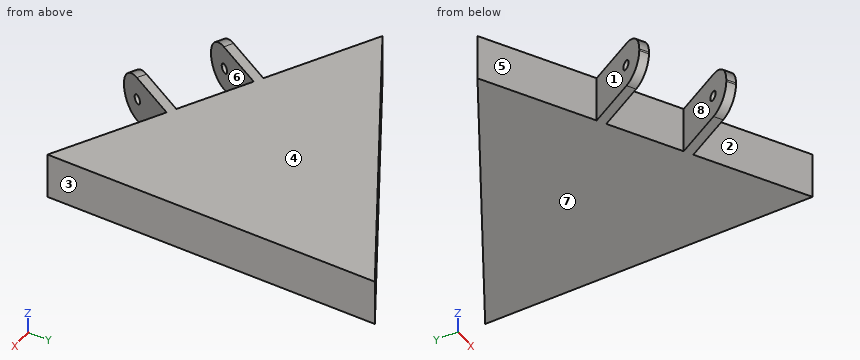
```python
from build123d import *

# Parameters (mm, degrees)
F1_DEPTH = 12.7
F2_W     = 2.54
F2_H     = 12.7
F3_DEPTH = 20.32
F4_R     = 1.27
F5_DEPTH = 39.1414
F6_R     = 6.096


with BuildPart() as f1:
    # F0 (on Top) → F1 (new body)
    with BuildSketch(Plane.XY):
        Polygon((25.4, -43.9940905122), (25.4, 43.9940905122), (-50.8, 0), align=None)
    extrude(amount=F1_DEPTH)

    # F2 (on face) → F3 (join)
    with BuildSketch(Plane(origin=(-12.7, -21.9970452561, 0), x_dir=(0.8660254038, -0.5, 0), z_dir=(-0.5, -0.8660254038, 0))):
        with Locations((11.43, 6.35)):
            Rectangle(F2_W, F2_H)
        with Locations((-11.43, 6.35)):
            Rectangle(F2_W, F2_H)
    extrude(amount=F3_DEPTH)

    # F4 (on face) → F5 (cut)
    with BuildSketch(Plane(origin=(10.9985226281, -6.35, 0), x_dir=(0.5, 0.8660254038, 0), z_dir=(0.8660254038, -0.5, 0))):
        with Locations((-39.37, 6.35)):
            Circle(F4_R)
    extrude(amount=-F5_DEPTH, mode=Mode.SUBTRACT)

    # F6
    f6_edges = [f1.edges().sort_by_distance(p)[0] for p in [
        (-32.75867, -33.879681, 0),
        (-32.75867, -33.879681, 12.7),
        (-12.96133, -45.309681, 12.7),
        (-12.96133, -45.309681, 0),
    ]]
    fillet(f6_edges, radius=F6_R)


solid = f1.part
```
The model under review builds one solid part; all positions refer to its coordinate system, in mm. Face numbers are marked on the shaded views. A direction names the side the tool comes from. Round coordinates to 2 decimals unless told otherwise and drop trailing zeros. Loops run counter-clockwise (first coordinate to the right, second up) from the corner with the lowest first, then second, coordinate; pieces in that order, holes last.
1) Clearance check with flat-ended pins moving along their axes: P1, Ø1.5, axis at y = -16.5, z = 4, coming from the -X side; P2, Ø5, axis at y = 25.5, z = 6.5, coming from the -X side; P3, Ø3, axis at x = -18, z = 5, coming from the +Y side. State where each tip first meets the part, or that it passes through.
Values follow:
P1: stops at x = -24.62
P2: stops at x = -10.96
P3: stops at y = 19.8
2) The part is to be moulded in two halves that separate along X. For the marked faces 1, 2, 3 and 4, say which applies: pulls with the +X half, pulls with the -X half, needs draft (parallel to the pull), parting line crosses it, or undercut.
Values follow:
face 1: pulls with the -X half
face 2: undercut
face 3: pulls with the +X half
face 4: needs draft
3) Tool access review of the marked faces 5, 6, 7 and 8: name each direction out of +Z, -Z, +X, -X, +Y, -Y from which nothing blocks a thin tool from reaching the whole face with its end or side.
Values follow:
face 5: +Z, -Z, -X
face 6: +Z, -Z, -Y
face 7: -Z, +X, -X, +Y, -Y
face 8: +Z, -Z
4) Consider section B-B on x = -6. State the section outline as (y, z) points.
Values follow:
outline: (-35.79, 0) - (-30.71, 0) - (-30.71, 12.7) - (-35.79, 12.7) - close; (-25.87, 0) - (25.87, 0) - (25.87, 12.7) - (-25.87, 12.7) - close
5) Wall thickness on line 1 along X through (y, z) = (-30, 3.5); line 2 along Y through (x, z) = (-12.5, 11); line 3 along X through (y, z) = (-30.5, 6.5): over which ranges is each line inside the solid? List them lowest first.
Values follow:
line 1: x = -31.99 to -29.05, -5.59 to -2.66, 1.16 to 25.4
line 2: y = -43.41 to -41.97, -22.11 to 22.11
line 3: x = -32.27 to -29.34, -5.88 to -2.94, 2.03 to 25.4
6) Consider section A-A on y = -25.5. State the section outline as (x, z) points, then the cut area to 3 significant figures.
Values follow:
outline: (-29.39, 0) - (-26.45, 0) - (-26.45, 12.7) - (-29.39, 12.7) - close; (-6.63, 0) - (25.4, 0) - (25.4, 12.7) - (-6.63, 12.7) - close
area: 444 mm2
7) Consider section D-D on x = 8. State the section outline as (y, z) points.
Values follow:
outline: (-33.95, 0) - (33.95, 0) - (33.95, 12.7) - (-33.95, 12.7) - close
8) Consider section C-C on z = 8.75. State the section outline as (x, y) points, then the cut area to 3 significant figures.
Values follow:
outline: (-50.8, 0) - (-23.7, -15.65) - (-33.66, -32.91) - (-31.46, -34.18) - (-21.5, -16.92) - (-3.9, -27.08) - (-13.87, -44.34) - (-11.67, -45.61) - (-1.7, -28.35) - (25.4, -43.99) - (25.4, 43.99) - close
area: 3,450 mm2
